Autodesk Inventor part; units mm, degrees
ref_plane "YZ Plane" through (0, 0, 0) normal (1, 0, 0) x (0, 1, 0)
ref_plane "XZ Plane" through (0, 0, 0) normal (0, 1, 0) x (-1, 0, 0)
ref_plane "XY Plane" through (0, 0, 0) normal (0, 0, 1) x (1, 0, 0)
sketch "スケッチ1" plane through (0, 0, 0) normal (0, 0, 1) x (1, 0, 0)
  circle A0 centre (0, 0) radius 9
  dimension "d0" = 18
extrude "押し出し1" add sketch "スケッチ1" along normal blind 2
sketch "スケッチ2" plane through (0, 0, 2) normal (0, 0, 1) x (1, 0, 0)
  circle A0 centre (0, 0) radius 3.5
  dimension "d3" = 7
extrude "押し出し2" add sketch "スケッチ2" along normal blind 2.5
sketch "スケッチ3" plane through (0, 0, 4.5) normal (0, 0, 1) x (1, 0, 0)
  circle A0 centre (0, 0) radius 2.2
  dimension "d6" = 4.4
extrude "押し出し3" cut sketch "スケッチ3" against normal blind 3.3
sketch "スケッチ4" plane through (0, 0, 1.2) normal (0, 0, 1) x (1, 0, 0)
  circle A0 centre (0, 0) radius 2.2
  circle A1 centre (0, 0) radius 1.15
  dimension "d9" = 2.3
extrude "押し出し4" cut sketch "スケッチ4" against normal through all contours A1
sketch "スケッチ5" plane through (0, 0, 0) normal (0, 0, -1) x (-1, 0, 0)
  circle A0 centre (0, 0) radius 6 construction
  line L0 (0, -11.2961) -> (0, 11.2961) construction
  line L1 (-11.4539, 0) -> (11.4539, 0) construction
  point P0 (0, 6)
  point P1 (-4.2426, 4.2426)
  point P2 (-6, 0)
  point P3 (-4.2426, -4.2426)
  point P4 (0, -6)
  point P5 (4.2426, -4.2426)
  point P6 (6, 0)
  point P7 (4.2426, 4.2426)
  dimension "d12" = 12
  dimension "d15" = 360
hole "穴1" at (0, 6, 0) at (4.2426, 4.2426, 0) at (6, 0, 0) at (4.2426, -4.2426, 0) at (0, -6, 0) at (-4.2426, -4.2426, 0) at (-6, 0, 0) at (-4.2426, 4.2426, 0) direction (0, 0, 1) diameter 1.567 end through all
properties part number "STS3032_Horn"
The listing builds one solid part. Answer for the finished solid, in the listing's coordinates (mm). A direction names the side the tool comes from. Coordinates: 2 decimals unless noted, no trailing zeros. Loops run counter-clockwise (first coordinate to the right, second up) from the corner with the lowest first, then second, coordinate; pieces in that order, holes last. Notation, with made-up numbers: (-1.5, -20.75) -> (48.5, -20.75) arc R23 cw to (48.5, -5.75) -> close; hole circle Ø4 at (62.5, -5.75). An arc over 180 degrees is marked (long way). Answer in a Markdown table with one row per item. Add a question column.
1. Consider line 1 (Y direction, x = 0, z = 1.25); line 2 (Y direction, x = 0.5, z = 0.5); line 3 (Z direction, x = 6, y = -1.75). Determine where each line is inside the solid, lowest interval first. Write a range as [from, to].
2. Flat-ended cylindrical pins translate along their axes: P1, Ø4, axis at x = 1, y = 4, coming from the +Z side; P2, Ø2, axis at x = 4.24, y = -4.24, coming from the +Z side; P3, Ø2, axis at x = 2, z = 0.5, coming from the +Y side; P4, Ø1.5, axis at y = 1.5, z = 1, coming from the +X side. Find the tip coordinate at first contact, or state that the pin passes through.
3. Determine the mould class of faces 3 (the flat face through (0, -2, 0)), 4 (the cylindrical face through (3.233, 1.341, 3.232)), 5 (the cylindrical face through (-3.48, 4.07, 1.01)), 6 (the cylindrical face through (-3.55, -3.88, 1.01)) for opening direction X: +X half, -X half, draft (parallel to the pull), parting line (faces both ways), or undercut.
4. The part is cut by section C-C, the plane x = -6. Write down the section's boundary in (y, z), then the cut area to 3 significant figures.
5. The part is cut by section A-A, the plane y = 0. Write down the section's boundary in (x, z).
6. For faces 1 (the cylindrical face through (0.3, 6.724, 1.014)), 2 (the flat face through (0, -4, 2)), determine the directions among +Z, -Z, +X, -X, +Y, -Y from which every point of the face is accessible in a straight line to the end or side of a thin tool.
Answer below:
| question | item | result |
|---|---|---|
| 1 | line 1 | [-9, -6.78], [-5.22, -2.2], [2.2, 5.22], [6.78, 9] |
| 1 | line 2 | [-8.99, -6.6], [-5.4, -1.04], [1.04, 5.4], [6.6, 8.99] |
| 1 | line 3 | [0, 2] |
| 2 | P1 | z = 4.5 |
| 2 | P2 | z = 2 |
| 2 | P3 | y = 8.94 |
| 2 | P4 | x = 8.97 |
| 3 | face 3 | draft |
| 3 | face 4 | parting line |
| 3 | face 5 | undercut |
| 3 | face 6 | undercut |
| 4 | outline | (-6.71, 0) -> (-0.78, 0) -> (-0.78, 2) -> (-6.71, 2) -> close; (0.78, 0) -> (6.71, 0) -> (6.71, 2) -> (0.78, 2) -> close |
| 4 | area | 23.7 mm2 |
| 5 | outline | (-9, 0) -> (-6.78, 0) -> (-6.78, 2) -> (-9, 2) -> close; (-5.22, 0) -> (-1.15, 0) -> (-1.15, 1.2) -> (-2.2, 1.2) -> (-2.2, 4.5) -> (-3.5, 4.5) -> (-3.5, 2) -> (-5.22, 2) -> close; (1.15, 0) -> (5.22, 0) -> (5.22, 2) -> (3.5, 2) -> (3.5, 4.5) -> (2.2, 4.5) -> (2.2, 1.2) -> (1.15, 1.2) -> close; (6.78, 0) -> (9, 0) -> (9, 2) -> (6.78, 2) -> close |
| 6 | face 1 | +Z, -Z |
| 6 | face 2 | +Z |
